```python
from build123d import *

# Parameters (mm, degrees)
F0_W     = 88.2142
F0_H     = 82.55
F1_DEPTH = 95.25
F2_W     = 44.1071
F2_H     = 82.55
F3_DEPTH = 82.55
F4_R     = 2.54
F5_R     = 2.413
F6_DEPTH = 19.05
F7_DEPTH = 127


with BuildPart() as f1:
    # F0 (on Front) → F1 (new body)
    with BuildSketch(Plane.XZ):
        with Locations((44.1071, 41.275)):
            Rectangle(F0_W, F0_H)
    extrude(amount=F1_DEPTH)

    # F2 (on face) → F3 (cut)
    with BuildSketch(Plane.XZ.offset(95.25)):
        with Locations((66.16065, 41.275)):
            Rectangle(F2_W, F2_H)
    extrude(amount=-F3_DEPTH, mode=Mode.SUBTRACT)

    # F4
    f4_edges = [f1.edges().sort_by_distance(p)[0] for p in [
        (44.1071, -95.25, 41.275),
        (88.2142, 0, 41.275),
        (88.2142, -12.7, 41.275),
        (0, -47.625, 0),
        (22.05355, -95.25, 0),
        (0, -95.25, 41.275),
        (22.05355, -95.25, 82.55),
        (0, -47.625, 82.55),
        (44.1071, 0, 82.55),
        (44.1071, -53.975, 82.55),
        (66.16065, -12.7, 82.55),
        (88.2142, -6.35, 82.55),
        (44.1071, -53.975, 0),
        (66.16065, -12.7, 0),
        (44.1071, 0, 0),
    ]]
    fillet(f4_edges, radius=F4_R)

    # F5 (on face) → F6 (cut)
    with BuildSketch(Plane.XZ.offset(95.25)):
        with BuildLine():
            ThreePointArc((27.813, 6.2865), (25.4, 8.6995), (22.987, 6.2865))
            ThreePointArc((22.987, 6.2865), (25.4, 3.8735), (27.813, 6.2865))
        make_face()
        with Locations((25.4, 72.9615)):
            Circle(F5_R)
    extrude(amount=-F6_DEPTH, mode=Mode.SUBTRACT)

    # F5 (on face) → F7 (cut)
    with BuildSketch(Plane.XZ.offset(95.25)):
        with Locations((62.8142, 6.2865)):
            Circle(F5_R)
        with Locations((62.8142, 72.9615)):
            Circle(F5_R)
    extrude(amount=-F7_DEPTH, mode=Mode.SUBTRACT)


solid = f1.part
```
Check sheet for the modelled part. Datum: model origin and axes. Units: mm. A direction names the side the tool comes from. Round coordinates to 2 decimals unless told otherwise and drop trailing zeros. Order: outer loops, then holes, each group sorted by start corner. A loop starts at its lowest first (then second) coordinate and runs counter-clockwise, first axis right, second up. Notation, with made-up numbers: (-19.5, -32) - (-6.5, -32) arc R28 ccw to (-6.5, -13) - close; hole circle Ø2 at (71.25, 10.25). An arc over 180 degrees is marked (long way). Answer as CSV lines item,"result". Start each with the question number.
1) Scan lines: probe 1 along Z at (x, y) = (25.4, -80); probe 2 along Y at (x, z) = (59, 46.5); probe 3 along X at (y, z) = (-85, 53). Record each from-to range of solid material in increasing order.
2) Section check B-B (z = 22). Record the cut outline in (x, y).
3) Depth check by flat-ended pin: pin 1 (3 mm diameter, centred on x = 25.4, z = 6.29, fed in from -Y); pin 2 (21 mm diameter, centred on x = 70, z = 35, fed in from -Y). Enter the tip coordinate at first touch or a pass-through.
4) Tool access check on faces 4 (the face through (24.9, -85.9, 70.6)), 5 (the face through (43.34, -50.86, 81.83)), 6 (the face through (44.107, -53, 41)). Record the directions out of +Z, -Z, +X, -X, +Y, -Y that give a thin tool (end or side, any length) a straight path to the whole face; none if there is none.
5) Section check A-A (x = 25.4). Record the cut outline in (y, z), then the cut area to 3 significant figures.
6) Section check C-C (y = -40). Record the cut outline in (x, z), then the cut area to 3 significant figures.
7) Draft check along Z on faces 1 (the face through (25, -47, 82.55)), 2 (the face through (65, -12.7, 42)), 3 (the face through (27.81, -85.86, 6.18)). Enter one of: +Z half, -Z half, draft (parallel to the pull), parting line (faces both ways), or undercut.
8) Section check D-D (y = -86). Record the cut outline in (x, z).
Determined:
1,probe 1,"0 to 3.87, 8.7 to 70.55, 75.37 to 82.55"
1,probe 2,"-12.7 to 0"
1,probe 3,"0 to 44.11"
2,outline,"(0, -92.71) arc R2.54 ccw to (2.54, -95.25) - (41.57, -95.25) arc R2.54 ccw to (44.11, -92.71) - (44.11, -12.7) - (85.67, -12.7) arc R2.54 ccw to (88.21, -10.16) - (88.21, -2.54) arc R2.54 ccw to (85.67, 0) - (0, 0) - close"
3,pin 1,"y = -76.2"
3,pin 2,"y = -12.7"
4,face 4,"-Y"
4,face 5,"+Z, +X, -Y"
4,face 6,"+Z, -Z, +X, -Y"
5,outline,"(-95.25, 2.54) arc R2.54 ccw to (-92.71, 0) - (-2.54, 0) arc R2.54 ccw to (0, 2.54) - (0, 80.01) arc R2.54 ccw to (-2.54, 82.55) - (-92.71, 82.55) arc R2.54 ccw to (-95.25, 80.01) - (-95.25, 75.37) - (-76.2, 75.37) - (-76.2, 70.55) - (-95.25, 70.55) - (-95.25, 8.7) - (-76.2, 8.7) - (-76.2, 3.87) - (-95.25, 3.87) - close"
5,area,"7,670 mm^2"
6,outline,"(0, 2.54) arc R2.54 ccw to (2.54, 0) - (41.57, 0) arc R2.54 ccw to (44.11, 2.54) - (44.11, 80.01) arc R2.54 ccw to (41.57, 82.55) - (2.54, 82.55) arc R2.54 ccw to (0, 80.01) - close"
6,area,"3,640 mm^2"
7,face 1,"+Z half"
7,face 2,"draft"
7,face 3,"undercut"
8,outline,"(0, 2.54) arc R2.54 ccw to (2.54, 0) - (41.57, 0) arc R2.54 ccw to (44.11, 2.54) - (44.11, 80.01) arc R2.54 ccw to (41.57, 82.55) - (2.54, 82.55) arc R2.54 ccw to (0, 80.01) - close; hole circle Ø4.83 at (25.4, 6.29); hole circle Ø4.83 at (25.4, 72.96)"
